Can you work these out from the model? Positions are in its coordinate system, mm. Face numbers are marked on the shaded views. A direction names the side the tool comes from. Coordinates: 2 decimals unless noted, no trailing zeros. Order: outer loops, then holes, each group sorted by start corner. A loop starts at its lowest first (then second) coordinate and runs counter-clockwise, first axis right, second up. Notation, with made-up numbers: M 88,-34 L 135,-34 A19 ccw 135,-25 Z; hole C 44.5,66.25 d2. An arc over 180 degrees is marked long. Answer as a JSON object with one key per item and string values.
from build123d import *

# Parameters (mm, degrees)
BOSS_EXTRUDE1_DEPTH = 3.175
SKETCH2_R           = 6.35
SKETCH2_R_2         = 3.175
BOSS_EXTRUDE2_DEPTH = 12.7
FILLET1_R           = 2.54
SKETCH3_R           = 3.175
BOSS_EXTRUDE3_DEPTH = 12.7


with BuildPart() as part:
    # Sketch1 → Boss-Extrude1 (new body)
    with BuildSketch(Plane(origin=(0, 0, 0), x_dir=(1, 0, 0), z_dir=(0, 1, 0))):
        Polygon((0, 9.953217651), (-12.7, 9.953217651), (-12.7, 16.303217651), (-25.4, 16.303217651), (-25.4, 9.096782349), (-25.4, -9.096782349), (25.4, -9.096782349), (25.4, 9.953217651), (12.7, 9.953217651), (12.7, 16.303217651), (0, 16.303217651), align=None)
    extrude(amount=BOSS_EXTRUDE1_DEPTH)

    # Sketch2 → Boss-Extrude2 (add)
    with BuildSketch(Plane(origin=(0, 0, 0), x_dir=(0, 0, -1), z_dir=(1, 0, 0))):
        with Locations((16.303217651, 6.35)):
            Circle(SKETCH2_R)
        with Locations((16.303217651, 6.35)):
            Circle(SKETCH2_R_2, mode=Mode.SUBTRACT)
    extrude(amount=BOSS_EXTRUDE2_DEPTH)

    # Fillet1
    fillet1_edges = [part.edges().sort_by_distance(p)[0] for p in [
        (25.4, 1.5875, 9.096782349),
        (-25.4, 1.5875, 9.096782349),
    ]]
    fillet(fillet1_edges, radius=FILLET1_R)

    # Sketch3 → Boss-Extrude3 (add)
    with BuildSketch(Plane.ZY.offset(25.4)):
        with BuildLine():
            Line((-16.303217651, 0), (-9.953217651, 0))
            Line((-9.953217651, 0), (-9.953217651, 3.175))
            Line((-9.953217651, 3.175), (-10.803956337, 3.175))
            ThreePointArc((-10.803956337, 3.175), (-19.478217651, 11.849261314), (-16.303217651, 0))
        make_face()
        with Locations((-16.303217651, 6.35)):
            Circle(SKETCH3_R, mode=Mode.SUBTRACT)
    extrude(amount=-BOSS_EXTRUDE3_DEPTH)


solid = part.part
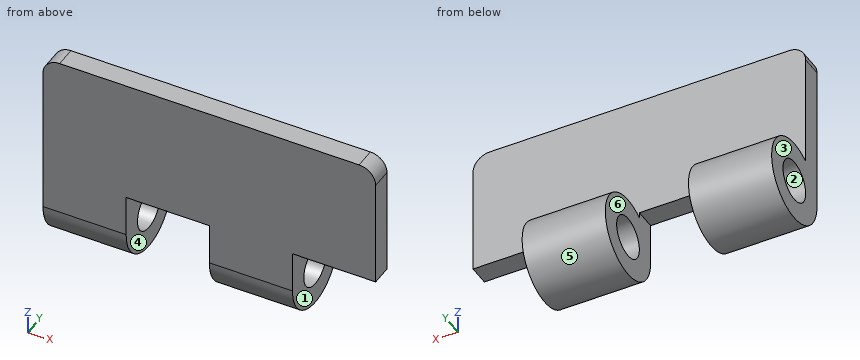
Item 1: I'm going to push flat-ended pins straight in: pin 1 (4 mm diameter, centred on y = 6.5, z = -19, fed in from +X); pin 2 (2.5 mm diameter, centred on x = -5.5, y = 1.5, fed in from -Z); pin 3 (1 mm diameter, centred on x = 1.5, y = 8.5, fed in from +Z). Where does each tip first touch, or does it pass through?
Answers follow:
{"pin 1": "stops at x = 12.7", "pin 2": "stops at z = -9.95", "pin 3": "stops at z = -10.17"}
Item 2: Please list where these lines run through material, in increasing order: line 1 (Z direction, x = -17, y = 6.35); line 2 (X direction, y = 7.5, z = -11.5); line 3 (Y direction, x = 18, z = 2) (3 decimals).
Answers follow:
{"line 1": "z = -22.65 to -19.48, -13.13 to -9.95", "line 2": "x = -25.4 to -12.7, 0 to 12.7", "line 3": "y = 0 to 3.175"}
Item 3: I want a section at C-C, the plane x = -14.5. Write out the boundary of the cut face in (y, z) (3 decimals), plus the area to 3 significant figures.
Answers follow:
{"outline": "M 0,-16.303 A6.35 ccw long 3.175,-10.804 L 3.175,9.097 L 0,9.097 Z; hole C 6.35,-16.303 d6.35", "area": "163 mm^2"}
Item 4: I want a section at D-D, the plane y = 10.25. Write out the boundary of the cut face in (x, z), plus the area to 3 significant figures.
Answers follow:
{"outline": "M -25.4,-21.31 L -12.7,-21.31 L -12.7,-11.29 L -25.4,-11.29 Z; M 0,-21.31 L 12.7,-21.31 L 12.7,-11.29 L 0,-11.29 Z", "area": "255 mm^2"}
Item 5: Which directions (+Z, -Z, +X, -X, +Y, -Y) give clear straight access to the entire face, cutting with the end or side of a thin tool? Please do the marked faces 1 and 2.
Answers follow:
{"face 1": "-Z, +X, +Y, -Y", "face 2": "+X, -X"}
Item 6: I want a section at A-A, the plane y = 6.35. Write out the boundary of the cut face in (x, z), plus the area to 3 significant figures.
Answers follow:
{"outline": "M -25.4,-22.65 L -12.7,-22.65 L -12.7,-19.48 L -25.4,-19.48 Z; M -25.4,-13.13 L -12.7,-13.13 L -12.7,-9.95 L -25.4,-9.95 Z; M 0,-22.65 L 12.7,-22.65 L 12.7,-19.48 L 0,-19.48 Z; M 0,-13.13 L 12.7,-13.13 L 12.7,-9.95 L 0,-9.95 Z", "area": "161 mm^2"}
Item 7: I want a section at B-B, the plane z = -15. Write out the boundary of the cut face in (x, y).
Answers follow:
{"outline": "M -25.4,0 L -12.7,0 L -12.7,3.45 L -25.4,3.45 Z; M -25.4,9.25 L -12.7,9.25 L -12.7,12.56 L -25.4,12.56 Z; M 0,0 L 12.7,0 L 12.7,3.45 L 0,3.45 Z; M 0,9.25 L 12.7,9.25 L 12.7,12.56 L 0,12.56 Z"}
Item 8: If we mould it in two halves opening along X, with no side actions, what happens to the marked faces 3, 4, 5 and 6? For each: pulls with the +X half, pulls with the -X half, needs draft (parallel to the pull), parting line crosses it, or undercut.
Answers follow:
{"face 3": "pulls with the -X half", "face 4": "undercut", "face 5": "needs draft", "face 6": "undercut"}
